from build123d import *

# Parameters (mm, degrees)
SKETCH1_W            = 69.5
SKETCH1_H            = 33.25
BOSS_EXTRUDE1_DEPTH  = 2.75
SKETCH2_W            = 33.25
SKETCH2_H            = 49
BOSS_EXTRUDE2_DEPTH  = 2.5
M3_CLEARANCE_HOLE1_D = 3.4


with BuildPart() as part:
    # Sketch1 → Boss-Extrude1 (new body)
    with BuildSketch(Plane(origin=(0, 0, 0), x_dir=(1, 0, 0), z_dir=(0, 1, 0))):
        with Locations((31.075, 14.125)):
            Rectangle(SKETCH1_W, SKETCH1_H)
    extrude(amount=BOSS_EXTRUDE1_DEPTH)

    # Sketch2 → Boss-Extrude2 (add)
    with BuildSketch(Plane.ZY.offset(3.675)):
        with Locations((-14.125, 24.5)):
            Rectangle(SKETCH2_W, SKETCH2_H)
    extrude(amount=BOSS_EXTRUDE2_DEPTH)

    # M3 Clearance Hole1 (through all)
    with Locations(Plane.ZY.offset(6.175)):
        with Locations((-5.8125, 5)):
            Hole(M3_CLEARANCE_HOLE1_D / 2)


solid = part.part
Here's how the part is built. I have some questions about the finished solid (model axes, mm). A direction names the side the tool comes from. Give positions to 0.01 mm unless a question says otherwise; leave off trailing zeros. Write each loop counter-clockwise with the first axis right and the second up, starting at its lowest first coordinate (ties: lowest second). Pieces come first, ordered by that corner, then holes. Notation, with made-up numbers: (63, -24) -> (111, -24) arc R22 cw to (111, -14) -> close; hole circle Ø6 at (87.25, 76). An arc over 180 degrees is marked (long way). Use one line per item in the form item = value. Start each with the question number.
1. Thinking about a two-plate mould opening in Y: for faces 1 (the face through (-5, 49, -14)), 2 (the face through (30, 0, -14)), 3 (the face through (-4.91, 3.34, -5.44)), 4 (the face through (65.825, 1, -14)), which applies, +Y half, -Y half, draft (parallel to the pull), parting line (faces both ways), or undercut?
2. On a 3-axis mill with a long thin cutter (end or side, diameter ignored), from which of +Z, -Z, +X, -X, +Y, -Y can I reach the whole of each face in a straight line? I mean faces 5 (the face through (-3.675, 26, -14)), 6 (the face through (19, 1, 2.5)). Say none if no direction works.
3. Imagine slicing it at D-D on y = 14.5. List the corners of the cut face in (x, z) for me (3 decimals), plus the area to 3 significant figures.
4. If I drill on L1, parallel to Y at x = 41, z = -9.5; L2, parallel to X at y = 27, z = -12.5 (3 decimals), over which ranges is the centre line in solid material (lowest first)?
5. Will these pins go through, and if not, where does the flat tip stop? pin 1 Ø12 at (y, z) = (28.5, -5) entering from +X (3 decimals); pin 2 Ø2 at (y, z) = (5, -5.81) entering from -X.
6. Imagine slicing it at B-B on z = -10.5. List the corners of the cut face in (x, y) for me (3 decimals), plus the area to 3 significant figures.
7. Imagine slicing it at C-C on x = 32. List the corners of the cut face in (y, z) for me, plus the area to 3 significant figures.
Entries:
q1.face_1 = +Y half
q1.face_2 = -Y half
q1.face_3 = undercut
q1.face_4 = draft
q2.face_5 = +Z, -Z, +X, +Y
q2.face_6 = +Z, +X, -X, +Y, -Y
q3.outline = (-6.175, -30.75) -> (-3.675, -30.75) -> (-3.675, 2.5) -> (-6.175, 2.5) -> close
q3.area = 83.1 mm²
q4.L1 = 0 to 2.75
q4.L2 = -6.175 to -3.675
q5.pin_1 = -3.675
q5.pin_2 = through
q6.outline = (-6.175, 0) -> (65.825, 0) -> (65.825, 2.75) -> (-3.675, 2.75) -> (-3.675, 49) -> (-6.175, 49) -> close
q6.area = 314 mm²
q7.outline = (0, -30.75) -> (2.75, -30.75) -> (2.75, 2.5) -> (0, 2.5) -> close
q7.area = 91.4 mm²
